Model file for the job. Use its own axes, mm. A direction names the side the tool comes from. Give positions to 0.01 mm unless a question says otherwise; leave off trailing zeros. Order: outer loops, then holes, each group sorted by start corner. A loop starts at its lowest first (then second) coordinate and runs counter-clockwise, first axis right, second up. Notation, with made-up numbers: M -28.75,85.5 L -1.75,85.5 A20 ccw -1.75,120.5 Z; hole C 13,30.5 d8. An arc over 180 degrees is marked long. Return JSON: item names as keys, results as strings. Group by question number.
1. Wall check: probe 1 along X at (y, z) = (4.7, 0); probe 2 along Y at (x, z) = (10, -13); probe 3 along X at (y, z) = (-0.5, -2.5). Give the ranges that are in metal, low to high. Write a range as [from, to].
2. Pin check, flat tips, straight feed: pin 1 (11 mm diameter, centred on x = 5, z = 2, fed in from -Y); pin 2 (1.5 mm diameter, centred on x = -4.5, z = -15, fed in from -Y); pin 3 (1.5 mm diameter, centred on x = 7, y = 12, fed in from -Z). Stop position of each tip, or through.
3. Slice it at D-D on z = 11.5. List the corners of the cut face in (x, y), then the cut area to 3 significant figures.
4. Two-plate mould, pull along Z, no slides. Class faces 4 (the face through (-10, 14.1, 5)), 5 (the face through (-8, 3.5, 2)), 6 (the face through (-13.137, 10.957, 1.725)), 7 (the face through (-7.81, 5.33, -1.73)): released by +Z, released by -Z, zero draft, split by the parting line, or undercut.
5. Slice it at C-C on y = 13.25. List the corners of the cut face in (x, z).
6. 3-axis set-ups, long thin cutter, end or side, ignore diameter. For faces 1 (the face through (10, -3.5, 5)), 2 (the face through (-4, 7.9, 13)), 3 (the face through (-4, 0, 13)): which of +Z, -Z, +X, -X, +Y, -Y reach the whole face in a straight line?
7. Slice it at B-B on z = 0. List the corners of the cut face in (x, y).
8. Slice it at A-A on x = 0. List the corners of the cut face in (y, z), then the cut area to 3 significant figures.
from build123d import *

# Parameters (mm, degrees)
CROQUIS1_R              = 19.86
SALIENTE_EXTRUIR1_DEPTH = 7.9
CROQUIS2_R              = 8
CORTAR_EXTRUIR1_DEPTH   = 7.9
CROQUIS3_R              = 13.25
CROQUIS3_R_2            = 11
SALIENTE_EXTRUIR2_DEPTH = 6.2
SALIENTE_EXTRUIR3_START = 3.5
CROQUIS4_R              = 13.25
CROQUIS4_R_2            = 11
SALIENTE_EXTRUIR3_DEPTH = 3.5
CROQUIS5_R              = 11
CORTAR_EXTRUIR2_DEPTH   = 7
CORTAR_EXTRUIR3_START   = -7
CROQUIS6_R              = 11
CORTAR_EXTRUIR3_DEPTH   = 7


with BuildPart() as part:
    # Croquis1 → Saliente-Extruir1 (new body)
    with BuildSketch(Plane(origin=(0, 0, 0), x_dir=(1, 0, 0), z_dir=(0, 1, 0))):
        with Locations(Location((0, 0, 0), (0, 0, 270))):
            Circle(CROQUIS1_R)
    extrude(amount=SALIENTE_EXTRUIR1_DEPTH)

    # Croquis2 → Cortar-Extruir1 (cut)
    with BuildSketch(Plane(origin=(0, 7.9, 0), x_dir=(1, 0, 0), z_dir=(0, 1, 0))):
        with Locations(Location((0, 0, 0), (0, 0, 270))):
            Circle(CROQUIS2_R)
    extrude(amount=-CORTAR_EXTRUIR1_DEPTH, mode=Mode.SUBTRACT)

    # Croquis3 → Saliente-Extruir2 (add)
    with BuildSketch(Plane(origin=(0, 7.9, 0), x_dir=(1, 0, 0), z_dir=(0, 1, 0))):
        with Locations(Location((0, 0, 0), (0, 0, 90))):
            Circle(CROQUIS3_R)
        with Locations(Location((0, 0, 0), (0, 0, 90))):
            Circle(CROQUIS3_R_2, mode=Mode.SUBTRACT)
    extrude(amount=SALIENTE_EXTRUIR2_DEPTH)

    # Croquis4 → Saliente-Extruir3 (add)
    with BuildSketch(Plane.XZ.offset(SALIENTE_EXTRUIR3_START)):
        with Locations(Location((0, 0, 0), (0, 0, 270))):
            Circle(CROQUIS4_R)
        with Locations(Location((0, 0, 0), (0, 0, 270))):
            Circle(CROQUIS4_R_2, mode=Mode.SUBTRACT)
    extrude(amount=-SALIENTE_EXTRUIR3_DEPTH)

    # Croquis5 → Cortar-Extruir2 (cut)
    with BuildSketch(Plane.XZ.offset(3.5)):
        with Locations(Location((0, 0, 0), (0, 0, 270))):
            Circle(CROQUIS5_R)
    extrude(amount=-CORTAR_EXTRUIR2_DEPTH, mode=Mode.SUBTRACT)

    # Croquis6 → Cortar-Extruir3 (cut)
    with BuildSketch(Plane(origin=(0, 14.1, 0), x_dir=(1, 0, 0), z_dir=(0, 1, 0)).offset(CORTAR_EXTRUIR3_START)):
        with Locations(Location((0, 0, 0), (0, 0, 90))):
            Circle(CROQUIS6_R)
    extrude(amount=CORTAR_EXTRUIR3_DEPTH, mode=Mode.SUBTRACT)


solid = part.part
Result:
{
 "1": {"probe 1": "x = [-19.86, -8], [8, 19.86]", "probe 2": "y = [0, 7.9]", "probe 3": "x = [-13.01, -10.71], [10.71, 13.01]"},
 "2": {"pin 1": "stops at y = 3.5", "pin 2": "stops at y = 0", "pin 3": "stops at z = -11.68"},
 "3": {"outline": "M -16.19,0 L -6.58,0 L -6.58,-3.5 L 6.58,-3.5 L 6.58,0 L 16.19,0 L 16.19,7.9 L 6.58,7.9 L 6.58,14.1 L -6.58,14.1 L -6.58,7.9 L -16.19,7.9 Z", "area": "384 mm2"},
 "4": {"face 4": "zero draft", "face 5": "undercut", "face 6": "split by the parting line", "face 7": "undercut"},
 "5": {"outline": "C 0,0 d26.5; hole C 0,0 d22"},
 "6": {"face 1": "+Z, -Z, +X, -X, -Y", "face 2": "+Y", "face 3": "-Y"},
 "7": {"outline": "M -19.86,0 L -13.25,0 L -13.25,-3.5 L -11,-3.5 L -11,3.5 L -8,3.5 L -8,7.1 L -11,7.1 L -11,14.1 L -13.25,14.1 L -13.25,7.9 L -19.86,7.9 Z; M 8,3.5 L 11,3.5 L 11,-3.5 L 13.25,-3.5 L 13.25,0 L 19.86,0 L 19.86,7.9 L 13.25,7.9 L 13.25,14.1 L 11,14.1 L 11,7.1 L 8,7.1 Z"},
 "8": {"outline": "M -3.5,-13.25 L 0,-13.25 L 0,-19.86 L 7.9,-19.86 L 7.9,-13.25 L 14.1,-13.25 L 14.1,-11 L 7.1,-11 L 7.1,-8 L 3.5,-8 L 3.5,-11 L -3.5,-11 Z; M -3.5,11 L 3.5,11 L 3.5,8 L 7.1,8 L 7.1,11 L 14.1,11 L 14.1,13.25 L 7.9,13.25 L 7.9,19.86 L 0,19.86 L 0,13.25 L -3.5,13.25 Z", "area": "205 mm2"}
}
